Check sheet for the drawn part. Datum: minimum x, y, z corner. Units: mm. A direction names the side the tool comes from. Give positions to 0.01 mm unless a question says otherwise; leave off trailing zeros. Write each loop counter-clockwise with the first axis right and the second up, starting at its lowest first coordinate (ties: lowest second). Pieces come first, ordered by that corner, then holes. Notation, with made-up numbers: (81.25, -2) - (117.25, -2) arc R12 ccw to (117.25, 5) - close; hole circle Ø8 at (47, 78). An arc over 180 degrees is marked (long way). One line per question, with ' | ' between items. Start each with the question number.
Q1. Section check D-D on x = 68. Record the boundary of the cut face in (y, z), and give its area (3 significant figures).
Q2. Section check B-B on y = 6. Record the boundary of the cut face in (x, z), and give its area (3 significant figures).
Q3. Gauge pin test, flat ends, axial feed: P1, Ø5, axis at x = 265.5, z = 130.5, coming from the +Y side; P2, Ø1, axis at y = 25.5, z = 77.5, coming from the +X side; P3, Ø3, axis at y = 2.5, z = 106.5, coming from the +X side. Record the tip position at first contact, or that the pin passes through.
Q4. Section check A-A on x = 248.5. Record the boundary of the cut face in (y, z).
Q5. Set-up check for the marked faces 1 and 2: record each of +Z, -Z, +X, -X, +Y, -Y from which the full face is reachable in a straight line by a thin tool's end or side.
Q6. Section check C-C on z = 149. Record the boundary of the cut face in (x, y).
Q7. Thickness scan on L1, parallel to X at y = 46, z = 141.5; L2, parallel to X at y = 7, z = 119; L3, parallel to Z at x = 242, y = 6. Record the ranges inside material, lowest first. Write a range as [from, to].
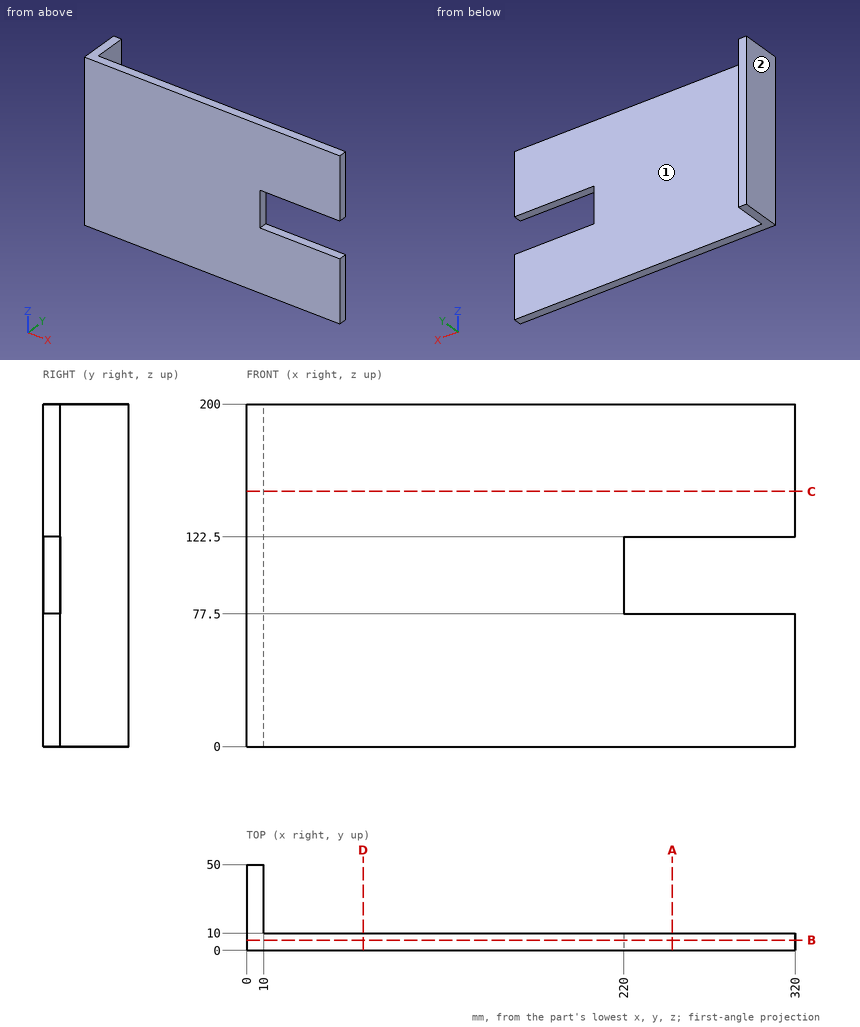
Working result:
1) outline: (0, 0) - (10, 0) - (10, 200) - (0, 200) - close | area: 2,000 mm2
2) outline: (0, 0) - (320, 0) - (320, 77.5) - (220, 77.5) - (220, 122.5) - (320, 122.5) - (320, 200) - (0, 200) - close | area: 59,500 mm2
3) P1: stops at y = 10 | P2: stops at x = 10 | P3: stops at x = 220
4) outline: (0, 0) - (10, 0) - (10, 77.5) - (0, 77.5) - close; (0, 122.5) - (10, 122.5) - (10, 200) - (0, 200) - close
5) face 1: +Z, -Z, +X, +Y | face 2: +Z, -Z, -X, +Y, -Y
6) outline: (0, 0) - (320, 0) - (320, 10) - (10, 10) - (10, 50) - (0, 50) - close
7) L1: x = [0, 10] | L2: x = [0, 220] | L3: z = [0, 77.5], [122.5, 200]
